The listing builds one solid part. Answer for the finished solid, in the listing's coordinates (mm). A direction names the side the tool comes from. Round coordinates to 2 decimals unless told otherwise and drop trailing zeros. Loops run counter-clockwise (first coordinate to the right, second up) from the corner with the lowest first, then second, coordinate; pieces in that order, holes last. Notation, with made-up numbers: M -16.5,-0.5 L 7.5,-0.5 A24 cw 7.5,22.5 Z; hole C 67,-9.5 d2. An arc over 180 degrees is marked long. Put each result on its own line as item: value. Start each with the question number.
(1) Straight lines are drawn through the part: line 1 (Z direction, x = -6.5, y = -2.75); line 2 (Y direction, x = 6.25, z = 14.5); line 3 (X direction, y = -6.75, z = 9). For each, find the intervals that lie inside material, in ascending order.
(2) Which of the six approach directions +Z, -Z, +X, -X, +Y, -Y give full straight-line access (tool end or side, diameter ignored) to faces 1 (the face through (-1.08, -4.88, 2.96)), 2 (the face through (5.2, 0.1, 20)), 3 (the face through (-1.73, -7.81, 12.9))?
(3) Flat-ended cylindrical pins translate along their axes: P1, Ø4, axis at y = 2, z = 14.5, coming from the +X side; P2, Ø3, axis at x = 3, z = 6.5, coming from the +Y side; P3, Ø5, axis at y = 3.5, z = 3, coming from the +X side; P4, Ø5, axis at y = -4, z = 20, coming from the -X side. Find the tip coordinate at first contact, or state that the pin passes through.
(4) Section A-A, the plane x = 0 is taken. Determine the outline of the cut face in (y, z), then the cut area to 3 significant figures.
(5) Section C-C, the plane z = 5.5 is taken. Determine the outline of the cut face in (x, y).
(6) Determine the mould class of faces 4 (the face through (5.2, 0.1, 6)), 5 (the face through (-1.08, -4.88, 22.96)), 6 (the face through (0, 0, 26)) for opening direction Z: released by +Z, released by -Z, zero draft, split by the parting line, or undercut.
(7) Section D-D, the plane z = 14 is taken. Determine the outline of the cut face in (x, y), then the cut area to 3 significant figures.
```python
from build123d import *

# Parameters (mm, degrees)
F0_R     = 5
F1_DEPTH = 6
F2_R     = 8
F2_R_2   = 5
F3_DEPTH = 14
F4_R     = 5
F5_DEPTH = 6


with BuildPart() as f1:
    # F0 (on Top) → F1 (new body)
    with BuildSketch(Plane.XY):
        Circle(F0_R)
    extrude(amount=F1_DEPTH)

    # F2 (on face) → F3 (join)
    with BuildSketch(Plane.XY.offset(6)):
        Circle(F2_R)
        Circle(F2_R_2, mode=Mode.SUBTRACT)
        Circle(F2_R_2)
    extrude(amount=F3_DEPTH)

    # F4 (on face) → F5 (join)
    with BuildSketch(Plane.XY.offset(20)):
        Circle(F4_R)
    extrude(amount=F5_DEPTH)


solid = f1.part
```
Recorded:
1. line 1: z = 6 to 20
1. line 2: y = -4.99 to 4.99
1. line 3: x = -4.29 to 4.29
2. face 1: -Z
2. face 2: +Z
2. face 3: +Z, -Z
3. P1: stops at x = 8
3. P2: stops at y = 7.86
3. P3: stops at x = 4.9
3. P4: stops at x = -7.86
4. outline: M -8,6 L -5,6 L -5,0 L 5,0 L 5,6 L 8,6 L 8,20 L 5,20 L 5,26 L -5,26 L -5,20 L -8,20 Z
4. area: 344 mm²
5. outline: C 0,0 d10
6. face 4: released by -Z
6. face 5: zero draft
6. face 6: released by +Z
7. outline: C 0,0 d16
7. area: 201 mm²
